from build123d import *

# Parameters (mm, degrees)
ESQUISSE1_R        = 2.5
ESQUISSE1_R_2      = 2.1
ESQUISSE1_R_3      = 1.6
BOSS_EXTRU_1_DEPTH = 3
BOSS_EXTRU_2_START = -3
ESQUISSE2_R        = 1.6
BOSS_EXTRU_2_DEPTH = 3


with BuildPart() as part:
    # Esquisse1 → Boss.-Extru.1 (new body)
    with BuildSketch(Plane.XY):
        with BuildLine():
            Line((-125, 15), (125, 15))
            ThreePointArc((125, 15), (140, 0), (125, -15))
            Line((125, -15), (-125, -15))
            ThreePointArc((-125, -15), (-140, 0), (-125, 15))
        make_face()
        with Locations((125, 0)):
            Circle(ESQUISSE1_R, mode=Mode.SUBTRACT)
        with Locations((-125, 0)):
            Circle(ESQUISSE1_R_2, mode=Mode.SUBTRACT)
        with Locations((125, 10)):
            Circle(ESQUISSE1_R_3, mode=Mode.SUBTRACT)
        with Locations(Location((125, -10, 0), (0, 0, 180))):
            Circle(ESQUISSE1_R_3, mode=Mode.SUBTRACT)
    extrude(amount=BOSS_EXTRU_1_DEPTH)

    # Esquisse2 → Boss.-Extru.2 (add)
    with BuildSketch(Plane.XY.offset(3).offset(BOSS_EXTRU_2_START)):
        with BuildLine():
            Line((140, 70), (110, 70))
            Line((110, 70), (110, 0))
            Line((110, 0), (122.5, 0))
            ThreePointArc((122.5, 0), (125, 2.5), (127.5, 0))
            Line((127.5, 0), (140, 0))
            Line((140, 0), (140, 70))
        make_face()
        with Locations((125, 10)):
            Circle(ESQUISSE2_R, mode=Mode.SUBTRACT)
    extrude(amount=BOSS_EXTRU_2_DEPTH)


solid = part.part
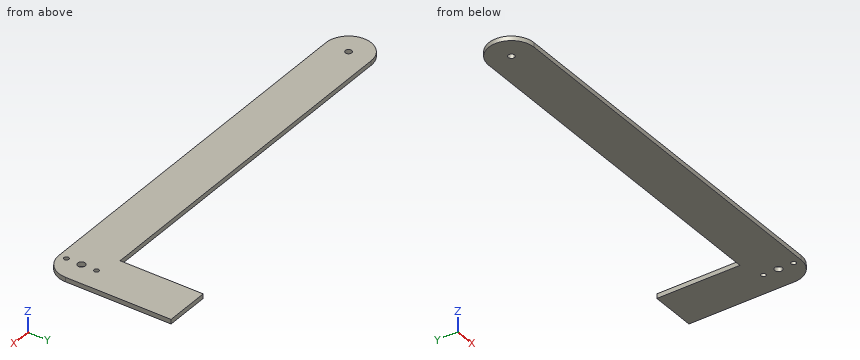
For this review, take the finished solid that the model builds, in its own axes (mm). Give positions to 0.01 mm unless a question says otherwise; leave off trailing zeros. Loops run counter-clockwise (first coordinate to the right, second up) from the corner with the lowest first, then second, coordinate; pieces in that order, holes last. Notation, with made-up numbers: (20, 0) -> (46, 0) arc R16 ccw to (46, 28) -> close; hole circle Ø3 at (-14, -11.5). An arc over 180 degrees is marked (long way). One line per question, with ' | ' between items.
1) We need section C-C (x = -74). Write out the cut boundary in (y, z).
Resolved:
outline: (-15, 0) -> (15, 0) -> (15, 3) -> (-15, 3) -> close
2) We need section A-A (z = 0.9). Write out the cut boundary in (x, y).
Resolved:
outline: (-125, -15) -> (125, -15) arc R15 ccw to (140, 0) -> (140, 70) -> (110, 70) -> (110, 15) -> (-125, 15) arc R15 ccw to start; hole circle Ø4.2 at (-125, 0); hole circle Ø5 at (125, 0); hole circle Ø3.2 at (125, -10); hole circle Ø3.2 at (125, 10)
3) To check wall thickness, follow probe 1 along Y at (x, z) = (125, 2.4); probe 2 along X at (y, z) = (41, 2.55); probe 3 along Y at (x, z) = (-125, 1.4). State the ranges of each line that lie inside material, in increasing order.
Resolved:
probe 1: y = -15 to -11.6, -8.4 to -2.5, 2.5 to 8.4, 11.6 to 70 | probe 2: x = 110 to 140 | probe 3: y = -15 to -2.1, 2.1 to 15
4) We need section B-B (y = 40). Write out the cut boundary in (x, z).
Resolved:
outline: (110, 0) -> (140, 0) -> (140, 3) -> (110, 3) -> close
5) Insertion check: pin 1 Ø2.5 at (x, y) = (-125, 0) entering from +Z; pin 2 Ø1.5 at (y, z) = (24.5, 2) entering from -X; pin 3 Ø3.5 at (x, y) = (125, 10) entering from +Z. Each pin has a flat end and moves straight along its axis. Give the tip position at first contact, or say it passes through.
Resolved:
pin 1: passes through | pin 2: stops at x = 110 | pin 3: stops at z = 3
